The listing builds one solid part. Answer for the finished solid, in the listing's coordinates (mm). A direction names the side the tool comes from. Coordinates: 2 decimals unless noted, no trailing zeros. Order: outer loops, then holes, each group sorted by start corner. A loop starts at its lowest first (then second) coordinate and runs counter-clockwise, first axis right, second up. Notation, with made-up numbers: (9.25, 29) -> (49.25, 29) arc R24 cw to (49.25, 47) -> close; hole circle Ø7 at (-40, 64). An arc over 180 degrees is marked (long way). Return JSON: item names as keys, results as strings.
from build123d import *

# Parameters (mm, degrees)
SKETCH020_R      = 1.5
EXTRUDE013_DEPTH = 100
SKETCH019_R      = 4
EXTRUDE012_DEPTH = 10
EXTRUDE014_DEPTH = 6.5
FILLET017_R      = 0.5
FILLET018_R      = 0.5


with BuildPart() as extrude013:
    # Sketch020 → Extrude013 (new body)
    with BuildSketch(Plane.YZ.offset(34.5)):
        with Locations((-7, -18.25)):
            Circle(SKETCH020_R)
        with Locations((7, -18.25)):
            Circle(SKETCH020_R)
    extrude(amount=-EXTRUDE013_DEPTH)


with BuildPart() as extrude012:
    # Sketch019 → Extrude012 (new body, symmetric)
    with BuildSketch(Plane.XY.offset(-20)):
        with Locations((26.625, 13.5)):
            Circle(SKETCH019_R)
        with Locations((26.625, -13.5)):
            Circle(SKETCH019_R)
    extrude(amount=EXTRUDE012_DEPTH, both=True)


with BuildPart() as extrude014:
    # Sketch022 → Extrude014 (new body)
    with BuildSketch(Plane(origin=(0, 0, -15), x_dir=(1, 0, 0), z_dir=(0, 0, -1))):
        Polygon((-22.5, 20.399377), (-22.5, -20.399423), (-34.5, -11.996933), (-34.5, 11.996887), align=None)
    extrude(amount=EXTRUDE014_DEPTH)


with BuildPart() as cut012:
    # Part__Mirroring001: instance of Extrude014
    add(extrude014.part.mirror(Plane(origin=(0, 0, 0), x_dir=(0, -1, 0), z_dir=(1, 0, 0))))

    # Cut011: cut Extrude012
    add(extrude012.part, mode=Mode.SUBTRACT)

    # Cut012: cut Extrude013
    add(extrude013.part, mode=Mode.SUBTRACT)


with BuildPart() as fillet017:
    # Sketch041 → Revolve003 (revolve)
    with BuildSketch(Plane.XZ):
        Polygon((22.625, -15), (22.625, -23.5), (24.025, -23.5), (25.025, -21.333333), (24.025, -21.333333), (25.025, -19.166667), (24.025, -19.166667), (25.025, -17), (25.625, -17), (25.625, -15), align=None)
    revolve(axis=Axis((26.625, 0, 0), (0, 0, 1)))


with BuildPart() as fillet017_1:
    # Revolve003 placement: moved
    add(fillet017.part.moved(Location((0, 13.5, 0))))

    # Fillet017
    fillet017_edges = [fillet017_1.edges().sort_by_distance(p)[0] for p in [
        (30.625, 13.5, -23.5),
    ]]
    fillet(fillet017_edges, radius=FILLET017_R)


with BuildPart() as fillet018:
    # Sketch042 → Revolve004 (revolve)
    with BuildSketch(Plane.XZ):
        Polygon((22.625, -15), (22.625, -23.5), (24.025, -23.5), (25.025, -21.333333), (24.025, -21.333333), (25.025, -19.166667), (24.025, -19.166667), (25.025, -17), (25.625, -17), (25.625, -15), align=None)
    revolve(axis=Axis((26.625, 0, 0), (0, 0, 1)))


with BuildPart() as fillet018_1:
    # Revolve004 placement: moved
    add(fillet018.part.moved(Location((0, 13.5, 0))))

    # Fillet018
    fillet018_edges = [fillet018_1.edges().sort_by_distance(p)[0] for p in [
        (30.625, 13.5, -23.5),
    ]]
    fillet(fillet018_edges, radius=FILLET018_R)


with BuildPart() as boden_tube_bracket_w_one_way_fitting:
    # Part__Mirroring002: instance of Fillet018
    add(fillet018_1.part.mirror(Plane(origin=(0, 0, 0), x_dir=(1, 0, 0), z_dir=(0, 1, 0))))

    # Fusion014: union Cut012, Fillet017
    add(cut012.part)
    add(fillet017_1.part)


solid = boden_tube_bracket_w_one_way_fitting.part
1. Each of these flat-tipped pins is pushed along its axis until it touches: pin 1 Ø3 at (x, z) = (25.5, -19) entering from +Y; pin 2 Ø3 at (x, y) = (26.625, -13.5) entering from -Z; pin 3 Ø2.5 at (y, z) = (-7, -18.25) entering from +X; pin 4 Ø2 at (x, z) = (27.5, -16.5) entering from +Y. Where does it stop, or does it pass through?
Answer block:
{"pin 1": "stops at y = 19.35", "pin 2": "stops at z = -17", "pin 3": "passes through", "pin 4": "stops at y = 17.6"}
2. The part is cut by section A-A on z = -18.25. Give the vertices of the cut face in (x, y) (3 decimals), and give its area (3 significant figures).
Answer block:
{"outline": "(22.5, -20.399) -> (26.641, -17.5) arc R4 ccw to (30.378, -14.883) -> (34.5, -11.997) -> (34.5, -8.5) -> (22.5, -8.5) -> close; (22.5, -5.5) -> (34.5, -5.5) -> (34.5, 5.5) -> (22.5, 5.5) -> close; (22.5, 8.5) -> (34.5, 8.5) -> (34.5, 11.997) -> (30.378, 14.883) arc R4 ccw to (26.641, 17.5) -> (22.5, 20.399) -> close; hole circle Ø4.354 at (26.625, -13.5); hole circle Ø4.354 at (26.625, 13.5)", "area": "291 mm2"}
3. Consider line 1 (Y direction, x = 26.75, z = -15.5); line 2 (Y direction, x = 23, z = -19); line 3 (Z direction, x = 28.5, y = 14). Determine where each line is inside the solid, lowest interval first. Write a range as from..to.
Answer block:
{"line 1": "y = -17.5..-14.49, -12.51..12.51, 14.49..17.5", "line 2": "y = -20.05..-8.3, -5.7..5.7, 8.3..20.05", "line 3": "z = -22.07..-21.33, -19.9..-19.17, -17.74..-15"}
4. Determine the mould class of faces 1 (the face through (28, 0, -15)), 2 (the face through (25, 14.2, -21.7)), 3 (the face through (25, 14.174, -17.346)) for opening direction Z: pulls with the +Z half, pulls with the -Z half, needs draft (parallel to the pull), parting line crosses it, or undercut.
Answer block:
{"face 1": "pulls with the +Z half", "face 2": "pulls with the -Z half", "face 3": "undercut"}
5. The part is cut by section B-B on y = -7. Give the vertices of the cut face in (x, z), and give its area (3 significant figures).
Answer block:
{"outline": "(22.5, -21.5) -> (34.5, -21.5) -> (34.5, -19.75) -> (22.5, -19.75) -> close; (22.5, -16.75) -> (34.5, -16.75) -> (34.5, -15) -> (22.5, -15) -> close", "area": "42.0 mm2"}
6. The part is cut by section C-C on z = -20.25. Give the vertices of the cut face in (x, y) (3 decimals).
Answer block:
{"outline": "(22.5, -20.399) -> (26.641, -17.5) arc R4 ccw to (30.378, -14.883) -> (34.5, -11.997) -> (34.5, 11.997) -> (30.378, 14.883) arc R4 ccw to (26.641, 17.5) -> (22.5, 20.399) -> close; hole circle Ø4.2 at (26.625, -13.5); hole circle Ø4.2 at (26.625, 13.5)"}
7. The part is cut by section D-D on y = -13.5. Give the vertices of the cut face in (x, z) (3 decimals).
Answer block:
{"outline": "(22.5, -21.5) -> (22.625, -21.5) -> (22.625, -23) arc R0.5 ccw to (23.125, -23.5) -> (24.025, -23.5) -> (25.025, -21.333) -> (24.025, -21.333) -> (25.025, -19.167) -> (24.025, -19.167) -> (25.025, -17) -> (25.625, -17) -> (25.625, -15) -> (22.5, -15) -> close; (27.625, -17) -> (28.225, -17) -> (29.225, -19.167) -> (28.225, -19.167) -> (29.225, -21.333) -> (28.225, -21.333) -> (29.225, -23.5) -> (30.125, -23.5) arc R0.5 ccw to (30.625, -23) -> (30.625, -21.5) -> (32.353, -21.5) -> (32.353, -15) -> (27.625, -15) -> close"}
8. For faces 4 (the face through (29.8, -15.93, -20.83)), 5 (the face through (25, -14.174, -17.346)), 6 (the face through (28.58, 5.89, -17.24)), determine the directions among +Z, -Z, +X, -X, +Y, -Y from which every point of the face is accessible in a straight line to the end or side of a thin tool.
Answer block:
{"face 4": "-Z", "face 5": "none", "face 6": "+X, -X"}
